Here's how the part is built. I have some questions about the finished solid (model axes, mm). Face numbers are marked on the shaded views. A direction names the side the tool comes from. Coordinates: 2 decimals unless noted, no trailing zeros. Write each loop counter-clockwise with the first axis right and the second up, starting at its lowest first coordinate (ties: lowest second). Pieces come first, ordered by that corner, then holes. Notation, with made-up numbers: (18, -37.75) - (63, -37.75) arc R11 cw to (63, -25.75) - close; hole circle Ø5 at (-37, -35.5). An arc over 180 degrees is marked (long way). Answer in a Markdown table with one row per item. Add a question column.
Item 1: If I drill on probe 1 along X at (y, z) = (9.8, 0); probe 2 along Z at (x, y) = (0, 3.7); probe 3 along X at (y, z) = (5, -1), over which ranges is the centre line in solid material (lowest first)? Write a range as from..to.
Item 2: Imagine slicing it at D-D (z = 0). State how many separate pieces and enclosed holes the cut face has, plus the area to 3 significant figures.
Item 3: I'm going to push flat-ended pins straight in: pin 1 (3 mm diameter, centred on x = 8.5, z = -0.5, fed in from -Y); pin 2 (5.5 mm diameter, centred on y = 8.5, z = 2, fed in from -X); pin 3 (5.5 mm diameter, centred on x = 25, z = 0, fed in from +Y); pin 4 (1 mm diameter, centred on y = 4, z = -1, fed in from -X). Where does each tip first touch, or does it pass through?
Item 4: Imagine slicing it at A-A (x = 45). Please give me the cut outline in (y, z), plus the area to 3 significant figures.
Item 5: Imagine slicing it at C-C (y = 7.25). Please give me the cut outline in (x, z).
Item 6: Which directions (+Z, -Z, +X, -X, +Y, -Y) give clear straight access to the entire face, cutting with the end or side of a thin tool? Please do the marked faces 4 and 5.
Item 7: Imagine slicing it at B-B (y = 3.5). Please give me the cut outline in (x, z).
Item 8: We'd pull the mould along X, two halves only. Please class the marked faces 1, 2 and 3: +X half, -X half, draft (parallel to the pull), parting line (faces both ways), or undercut.
Autodesk Inventor part; units mm, degrees
ref_plane "YZ Plane" through (0, 0, 0) normal (1, 0, 0) x (0, 1, 0)
ref_plane "XZ Plane" through (0, 0, 0) normal (0, 1, 0) x (-1, 0, 0)
ref_plane "XY Plane" through (0, 0, 0) normal (0, 0, 1) x (1, 0, 0)
sketch "Náčrt1" plane through (0, 0, 0) normal (0, 1, 0) x (-1, 0, 0)
  circle A0 centre (0, 0) radius 10
  line L0 (0, -10) -> (-50, -10)
  line L1 (-50, -10) -> (-50, 10)
  line L2 (-50, 10) -> (0, 10)
  circle A1 centre (0, 0) radius 3
  circle A2 centre (0, 0) radius 7.5 construction
  dimension "d0" = 6
  dimension "d1" = 15
  dimension "d2" = 20
  dimension "d3" = 50
extrude "Vysunutí1" add sketch "Náčrt1" along normal blind 6
sketch "Náčrt2" plane through (0, 6, 0) normal (0, 1, 0) x (1, 0, 0)
  line L0 (0, -10) -> (50, -10)
  line L1 (50, -10) -> (50, 10)
  line L2 (50, 10) -> (0, 10)
  arc A0 (0, 10) -> (0, -10) centre (0, 0) ccw
  circle A1 centre (0, 0) radius 3
  circle A2 centre (45, 0) radius 1.6
  circle A3 centre (25, 0) radius 1.6
  dimension "d6" = 5
  dimension "d7" = 25
  dimension "d8" = 3.2
extrude "Vysunutí2" cut sketch "Náčrt2" against normal through all contours A2 | A3
sketch "Náčrt5" plane through (0, 6, 0) normal (0, 1, 0) x (1, 0, 0)
  circle A0 centre (45, 0) radius 1.6
  circle A1 centre (25, 0) radius 1.6
  line L0 (0, -10) -> (50, -10)
  line L1 (50, -10) -> (50, 10)
  line L2 (50, 10) -> (0, 10)
  arc A2 (0, 10) -> (0, -10) centre (0, 0) ccw
  circle A3 centre (0, 0) radius 3
  line L3 (20, 10) -> (20, -10)
  dimension "d19" = 30
extrude "Vysunutí5" add sketch "Náčrt5" along normal blind 5 contours L3 L2 L1 L0
sketch "Náčrt7" plane through (0, 11, 0) normal (0, 1, 0) x (1, 0, 0)
  line L0 (50, 10) -> (20, 10)
  line L1 (20, 10) -> (20, -10)
  line L2 (20, -10) -> (50, -10)
  line L3 (50, -10) -> (50, 10)
  circle A0 centre (25, 0) radius 1.6
  circle A1 centre (45, 0) radius 1.6
  circle A2 centre (25, 0) radius 1.6
  circle A3 centre (25, 0) radius 3
  circle A4 centre (45, 0) radius 1.6
  circle A5 centre (45, 0) radius 3
  point P0 (0, 0)
  dimension "d22" = 6
extrude "Vysunutí6" cut sketch "Náčrt7" against normal blind 3 contours A3 | A5
sketch "Náčrt8" plane through (50, 0, 10) normal (1, 0, 0) x (0, 0, -1)
  line L0 (0, 0) -> (20, 0)
  line L1 (20, 0) -> (20, 11)
  line L2 (0, 11) -> (20, 11)
  line L3 (0, 0) -> (0, 11)
  point P0 (10, 0)
extrude "Vysunutí7" cut sketch "Náčrt8" against normal blind 0.5
chamfer "Zkosení2" distance 0.5 angle 45 20 edges at (20, 11, 0) (22, 11, 0) (42, 11, 0) (24.75, 0, 10) (-10, 0, 0) (24.75, 0, -10) (10, 6, 10) (-10, 6, 0) (10, 6, -10) (34.75, 11, 10) (49.5, 11, 0) (34.75, 11, -10) (49.5, 0, 0) (49.5, 5.5, 10) (49.5, 5.5, -10) (3, 6, 0) (20, 6, 0) (3, 0, 0) (23.4, 0, 0) (43.4, 0, 0)
properties part number "middle_joint"
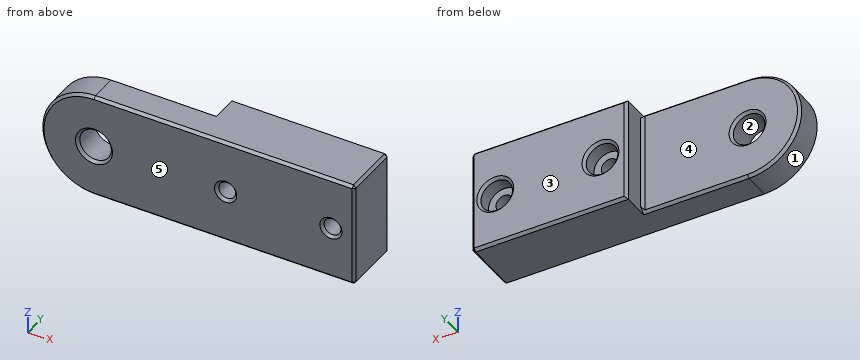
Here are the results:
| question | item | result |
|---|---|---|
| 1 | probe 1 | x = 20..22, 28..42, 48..49.5 |
| 1 | probe 2 | z = -10..-3, 3..10 |
| 1 | probe 3 | x = -9.95..-2.83, 2.83..23.75, 26.25..43.75, 46.25..49.5 |
| 2 | separate pieces | 4 |
| 2 | enclosed holes | 0 |
| 2 | area | 379 mm2 |
| 3 | pin 1 | stops at y = 0 |
| 3 | pin 2 | stops at x = -9.59 |
| 3 | pin 3 | stops at y = 8 |
| 3 | pin 4 | stops at x = -9.99 |
| 4 | outline | (0, -9.5) - (0.5, -10) - (10.5, -10) - (11, -9.5) - (11, -3.5) - (10.5, -3) - (8, -3) - (8, -1.6) - (0.5, -1.6) - (0, -2.1) - close; (0, 2.1) - (0.5, 1.6) - (8, 1.6) - (8, 3) - (10.5, 3) - (11, 3.5) - (11, 9.5) - (10.5, 10) - (0.5, 10) - (0, 9.5) - close |
| 4 | area | 175 mm2 |
| 5 | outline | (20, -10) - (49, -10) - (49.5, -9.5) - (49.5, 9.5) - (49, 10) - (20, 10) - close; hole circle Ø3.2 at (25, 0); hole circle Ø3.2 at (45, 0) |
| 6 | face 4 | +Z, -Z, -X, +Y |
| 6 | face 5 | +Z, -Z, +X, -X, -Y |
| 7 | outline | (0, -10) - (49, -10) - (49.5, -9.5) - (49.5, 9.5) - (49, 10) - (0, 10) arc R10 ccw to start; hole circle Ø6 at (0, 0); hole circle Ø3.2 at (25, 0); hole circle Ø3.2 at (45, 0) |
| 8 | face 1 | -X half |
| 8 | face 2 | undercut |
| 8 | face 3 | draft |
